from build123d import *

# Parameters (mm, degrees)
BOSS_EXTRU_1_DEPTH = 50


with BuildPart() as part:
    # Esquisse1 → Boss.-Extru.1 (new body)
    with BuildSketch(Plane.XY):
        with BuildLine():
            Line((69.091744654, -14.415915473), (70.48859579, 3.584084527))
            Line((70.48859579, 3.584084527), (69.908185058, 3.584084527))
            ThreePointArc((69.908185058, 3.584084527), (66.086740028, 23.076888708), (56.943655444, 40.711424744))
            ThreePointArc((56.943655444, 40.711424744), (49.968292573, 41.870869794), (48.808847523, 34.895506923))
            ThreePointArc((48.808847523, 34.895506923), (59.820145904, -4.642213263), (42.84093319, -42.007790271))
            ThreePointArc((42.84093319, -42.007790271), (42.910361767, -49.078517226), (49.981088722, -49.009088649))
            ThreePointArc((49.981088722, -49.009088649), (61.735305745, -32.996242584), (68.518282775, -14.32637168))
            Line((68.518282775, -14.32637168), (69.091744654, -14.415915473))
        make_face()
    extrude(amount=BOSS_EXTRU_1_DEPTH)


solid = part.part
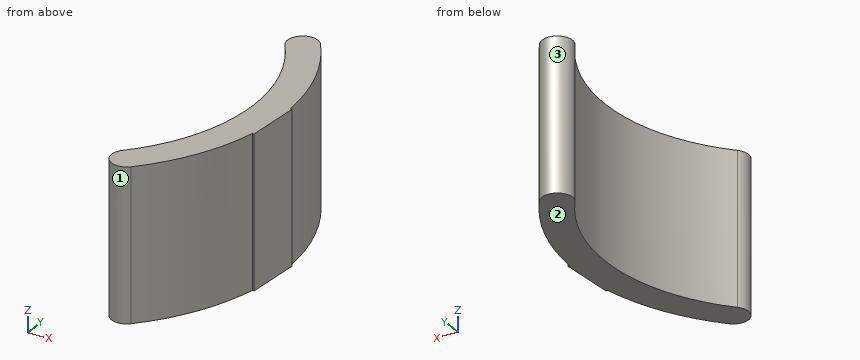
The listing builds one solid part. Answer for the finished solid, in the listing's coordinates (mm). Face numbers are marked on the shaded views. Coordinates: 2 decimals unless noted, no trailing zeros. Order: outer loops, then holes, each group sorted by start corner. A loop starts at its lowest first (then second) coordinate and runs counter-clockwise, first axis right, second up. Notation, with made-up numbers: (8.25, 67) -> (22.25, 67) arc R11 ccw to (22.25, 83) -> close; hole circle Ø10 at (-5.5, -15.75). An arc over 180 degrees is marked (long way). Answer in a Markdown table with one row per item. Add a question column.
Item 1: Find section A-A (x = 53.5). Write down the section's boundary in (y, z).
Item 2: Determine the mould class of the marked faces 1, 2 and 3 for opening direction Y: +Y half, -Y half, draft (parallel to the pull), parting line (faces both ways), or undercut.
Item 3: Each of these flat-tipped pins is pushed along its axis until it touches: P1, Ø2, axis at x = 60.5, z = 18.5, coming from the -Y side; P2, Ø1, axis at y = 8, z = 22, coming from the -X side; P3, Ø8, axis at y = -34.5, z = 38.5, coming from the -X side. Where does it stop, or does it pass through?
Item 4: Find section B-B (z = 43). Write down the section's boundary in (x, y).
Item 5: Find section C-C (x = 58). Write down the section's boundary in (y, z).
Item 6: Find the intervals of material crossed by L1, parallel to Y at x = 55.5, z = 4; L2, parallel to Y at x = 53, z = 39.5; L3, parallel to X at y = -11.5, z = 2, in increasing order. Write a range as from..to.
Item 7: Find section D-D (y = -8.5). Write down the section's boundary in (x, z), then the cut area to 3 significant figures.
Result set:
| question | item | result |
|---|---|---|
| 1 | outline | (-45.14, 0) -> (-27.16, 0) -> (-27.16, 50) -> (-45.14, 50) -> close; (27.16, 0) -> (42.76, 0) -> (42.76, 50) -> (27.16, 50) -> close |
| 2 | face 1 | parting line |
| 2 | face 2 | draft |
| 2 | face 3 | undercut |
| 3 | P1 | stops at y = -36.87 |
| 3 | P2 | stops at x = 59.39 |
| 3 | P3 | stops at x = 46.02 |
| 4 | outline | (42.84, -42.01) arc R5 ccw to (49.98, -49.01) arc R70 ccw to (68.52, -14.33) -> (69.09, -14.42) -> (70.49, 3.58) -> (69.91, 3.58) arc R70 ccw to (56.94, 40.71) arc R5 ccw to (48.81, 34.9) arc R60 cw to start |
| 5 | outline | (-39.19, 0) -> (-15.36, 0) -> (-15.36, 50) -> (-39.19, 50) -> close; (15.36, 0) -> (39.19, 0) -> (39.19, 50) -> (15.36, 50) -> close |
| 6 | L1 | y = -42.66..-22.8, 22.8..42.06 |
| 6 | L2 | y = -45.73..-28.12, 28.12..42.8 |
| 6 | L3 | x = 58.89..69.32 |
| 7 | outline | (59.39, 0) -> (69.55, 0) -> (69.55, 50) -> (59.39, 50) -> close |
| 7 | area | 508 mm² |
